For this review, take the finished solid that the model builds, in its own axes (mm). A direction names the side the tool comes from. Coordinates: 2 decimals unless noted, no trailing zeros. Loops run counter-clockwise (first coordinate to the right, second up) from the corner with the lowest first, then second, coordinate; pieces in that order, holes last. Notation, with made-up numbers: M 24,66.5 L 66,66.5 A18 cw 66,86.5 Z; hole C 82,47 d10. An arc over 180 degrees is marked long. Put each result on its own line as item: value.
```python
from build123d import *

# Parameters (mm, degrees)
F1_DEPTH = 50.8
F2_DEPTH = 25.4
F4_W     = 36.810688
F4_H     = 33.923566
F6_DEPTH = 117.714763
F7_DEPTH = 53.512752
F9_DEPTH = 50.799541


with BuildPart() as f1:
    # F0 (on Front) → F1 (new body)
    with BuildSketch(Plane.XZ):
        Polygon((37.712902, 42.765312), (-34.284458, 41.863091), (-34.284458, -46.374276), (37.712902, -46.374276), align=None)
    extrude(amount=-F1_DEPTH)

    # F1_face (on face) → F2 (join)
    with BuildSketch(Plane(origin=(1.775257, 50.8, -2.029655), x_dir=(1, 0, 0), z_dir=(0, 1, 0))):
        Polygon((-36.059715, -43.892746), (35.937644, -44.794967), (35.937644, 44.344621), (-36.059715, 44.344621), align=None)
    extrude(amount=F2_DEPTH)

    # F4 (on face) → F6 (join)
    with BuildSketch(Plane.XZ):
        with Locations((3.428448, 3.067523)):
            Rectangle(F4_W, F4_H)
    extrude(amount=-F6_DEPTH)

    # F4 (on face) → F7 (join)
    with BuildSketch(Plane.XZ):
        with Locations((3.428448, 3.067523)):
            Rectangle(F4_W, F4_H)
    extrude(amount=F7_DEPTH)

    # F8 (on face) → F9 (join)
    with BuildSketch(Plane.XZ.offset(53.512752)):
        Polygon((-14.976896, 20.029306), (0, 6.306419), (21.833792, -13.89426), (21.833792, 20.029306), align=None)
    extrude(amount=F9_DEPTH)


solid = f1.part
```
(1) Add section C-C (y = -20). Write out the cut boundary in (x, z).
Determined:
outline: M -14.98,-13.89 L 21.83,-13.89 L 21.83,20.03 L -14.98,20.03 Z
(2) For pin 1 (8 mm diameter, centred on x = -4, y = -56, fed in from +Z); pin 2 (5 mm diameter, centred on x = -17.5, z = -18.5, fed in from -Y); pin 3 (10 mm diameter, centred on x = -15, y = 75, fed in from +Z), all flat-tipped, find the tip position at first contact; note any pin that passes through.
Determined:
pin 1: stops at z = 20.03
pin 2: stops at y = 0
pin 3: stops at z = 42.17
(3) Add section B-B (x = -7). Write out the cut boundary in (y, z) (3 decimals).
Determined:
outline: M -104.312,12.72 L -53.513,12.72 L -53.513,-13.894 L 0,-13.894 L 0,-46.374 L 76.2,-46.374 L 76.2,-13.894 L 117.715,-13.894 L 117.715,20.029 L 76.2,20.029 L 76.2,42.205 L 0,42.205 L 0,20.029 L -104.312,20.029 Z
(4) Tool access review of faces 4 (the flat face through (4, -51, 20.029)), 5 (the flat face through (-14.977, 97, 3)), 6 (the flat face through (-1, -53.513, 0)), 7 (the flat face through (21.834, 97, 3)): name each direction out of +Z, -Z, +X, -X, +Y, -Y from which nothing blocks a thin tool from reaching the whole face with its end or side.
Determined:
face 4: +Z, +X, -X, -Y
face 5: +Z, -Z, -X, +Y
face 6: -Z, -X, -Y
face 7: +Z, -Z, +X, +Y
(5) Add section D-D (x = 11.5). Write out the cut boundary in (y, z), plus the area to 3 significant figures.
Determined:
outline: M -104.31,-4.33 L -53.51,-4.33 L -53.51,-13.89 L 0,-13.89 L 0,-46.37 L 76.2,-46.37 L 76.2,-13.89 L 117.71,-13.89 L 117.71,20.03 L 76.2,20.03 L 76.2,42.44 L 0,42.44 L 0,20.03 L -104.31,20.03 Z
area: 11,200 mm^2
(6) Draft analysis for pull direction Z (two halves, no side actions). For faces 1 (the flat face through (3, -26, -13.894)), 2 (the flat face through (3, 97, 20.029)), 3 (the flat face through (-14.977, -26, 3)), state which applies: +Z half, -Z half, draft (parallel to the pull), parting line (faces both ways), or undercut.
Determined:
face 1: -Z half
face 2: +Z half
face 3: draft
(7) Wall thickness on line 1 along X through (y, z) = (-20, 13); line 2 along Y through (x, z) = (-14, -38); line 3 along Z through (x, y) = (4, 89.5): over which ranges is each line inside the solid? List them lowest first. Write a range as [from, to].
Determined:
line 1: x = [-14.98, 21.83]
line 2: y = [0, 76.2]
line 3: z = [-13.89, 20.03]
